from build123d import *

# Parameters (mm, degrees)
SKETCH1_R           = 16
BOSS_EXTRUDE1_DEPTH = 8.5
SKETCH2_W           = 1
SKETCH2_H           = 0.1
CUT_EXTRUDE1_DEPTH  = 1


with BuildPart() as part:
    # Sketch1 → Boss-Extrude1 (new body)
    with BuildSketch(Plane(origin=(0, 0, 0), x_dir=(0, 0, -1), z_dir=(1, 0, 0))):
        Circle(SKETCH1_R)
    extrude(amount=BOSS_EXTRUDE1_DEPTH)

    # Sketch2 → Cut-Revolve1 (revolve, cut)
    with BuildSketch(Plane.XY, mode=Mode.PRIVATE) as cut_revolve1_sk:
        with Locations((8, 15.95)):
            Rectangle(SKETCH2_W, SKETCH2_H)
    revolve(cut_revolve1_sk.sketch.rotate(Axis((8.5, 0, 0), (-1, 0, 0)), 90), axis=Axis((8.5, 0, 0), (-1, 0, 0)), mode=Mode.SUBTRACT)

    # Sketch3 → Cut-Extrude1 (cut)
    with BuildSketch(Plane(origin=(8.5, 0, 0), x_dir=(0, 0, -1), z_dir=(1, 0, 0))):
        Polygon((-1, 15.814143289), (-1, 17.814143289), (1, 17.814143289), (1, 15.814143289), (1, 13.814143289), (-1, 13.814143289), align=None)
        Polygon((1, -17.814143289), (1, -15.814143289), (1, -13.814143289), (-1, -13.814143289), (-1, -15.814143289), (-1, -17.814143289), align=None)
    extrude(amount=-CUT_EXTRUDE1_DEPTH, mode=Mode.SUBTRACT)


solid = part.part
Here's how the part is built. I have some questions about the finished solid (model axes, mm). A direction names the side the tool comes from. Coordinates: 2 decimals unless noted, no trailing zeros. Write each loop counter-clockwise with the first axis right and the second up, starting at its lowest first coordinate (ties: lowest second). Pieces come first, ordered by that corner, then holes.
Item 1: I want a section at C-C on x = 4. Write out the boundary of the cut face in (y, z).
Item 2: If we mould it in two halves opening along Z, with no side actions, what happens to faces 4 (the cylindrical face through (8.007, -0.336, 15.896)), 5 (the flat face through (8, -15, 1)), 6 (the cylindrical face through (8.007, 0.336, -15.896))? For each: +Z half, -Z half, draft (parallel to the pull), parting line (faces both ways), or undercut.
Item 3: I want a section at B-B on z = 0. Write out the boundary of the cut face in (x, y), and give its area (3 significant figures).
Item 4: I want a section at A-A on x = 8. Write out the boundary of the cut face in (y, z).
Item 5: If I drill on line 1 (Z direction, x = 3.25, y = -0.5); line 2 (Y direction, x = 2, z = -2); line 3 (Y direction, x = 6.25, z = 0), over which ranges is the centre line in solid material (lowest first)?
Item 6: On a 3-axis mill with a long thin cutter (end or side, diameter ignored), from which of +Z, -Z, +X, -X, +Y, -Y can I reach the whole of each face in a straight line? I mean faces 1 (the flat face through (8, -13.814, 0)), 2 (the cylindrical face through (3.7, -15.62, 3.47)), 3 (the flat face through (8, 13.814, 0)). Say none if no direction works.
Item 7: Will these pins go through, and if not, where does the flat tip stop? pin 1 (1.1 mm diameter, centred on x = 8, y = -15, fed in from -Z); pin 2 (1.1 mm diameter, centred on x = 8, y = 14.5, fed in from +Z); pin 3 (1.5 mm diameter, centred on x = 3.5, z = -7, fed in from +Y); pin 4 (1.1 mm diameter, centred on x = 8, z = 0, fed in from -Y).
Findings below:
1. outline: circle Ø32 at (0, 0)
2. face 4: +Z half
2. face 5: undercut
2. face 6: -Z half
3. outline: (0, -16) - (7.5, -16) - (7.5, -13.81) - (8.5, -13.81) - (8.5, 13.81) - (7.5, 13.81) - (7.5, 16) - (0, 16) - close
3. area: 268 mm2
4. outline: (-15.87, -1) arc R15.9 ccw to (15.87, -1) - (13.81, -1) - (13.81, 1) - (15.87, 1) arc R15.9 ccw to (-15.87, 1) - (-13.81, 1) - (-13.81, -1) - close
5. line 1: z = -15.99 to 15.99
5. line 2: y = -15.87 to 15.87
5. line 3: y = -16 to 16
6. face 1: +X, -Y
6. face 2: +X, -X
6. face 3: +X, +Y
7. pin 1: stops at z = -6.63
7. pin 2: stops at z = 7.63
7. pin 3: stops at y = 14.73
7. pin 4: stops at y = -16
